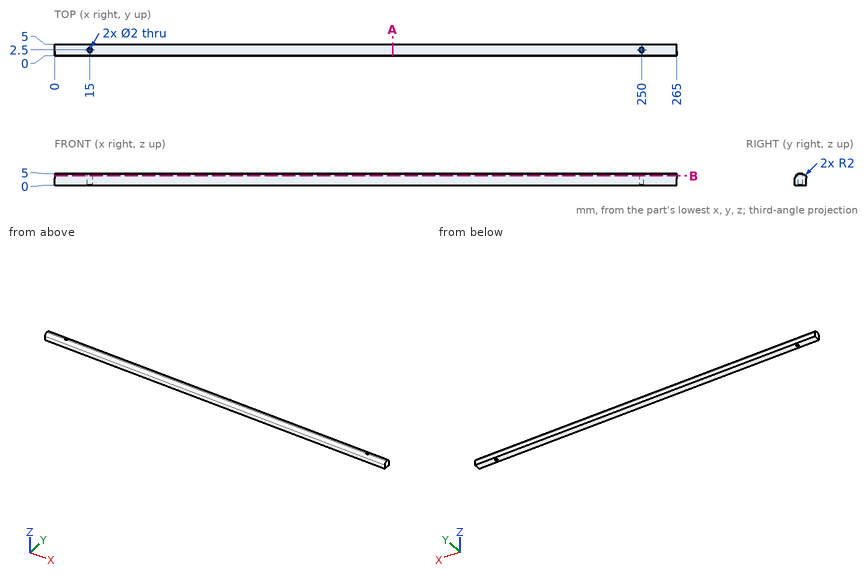
Study the drawing (mm; zero at the part's minimum x, y, z) and answer. Round coordinates to 2 decimals unless told otherwise and drop trailing zeros. Write each loop counter-clockwise with the first axis right and the second up, starting at its lowest first coordinate (ties: lowest second). Pieces come first, ordered by that corner, then holes. Notation, with made-up numbers: (15.5, 55.25) - (40.5, 55.25) arc R17 cw to (40.5, 65.25) - close; hole circle Ø7 at (56.25, 84.5). An arc over 180 degrees is marked (long way). Use CSV: the item, a comma, the result in double quotes.
Q1. Find section B-B, the plane z = 4.1. Write down the section's boundary in (x, y).
Values:
outline,"(0, 0.33) - (265, 0.33) - (265, 4.67) - (0, 4.67) - close; hole circle Ø2 at (15, 2.5); hole circle Ø2 at (250, 2.5)"
Q2. Find section A-A, the plane x = 144. Write down the section's boundary in (y, z), then the cut area to 3 significant figures.
Values:
outline,"(0, 0) - (5, 0) - (5, 3) arc R2 ccw to (3, 5) - (2, 5) arc R2 ccw to (0, 3) - close"
area,"23.3 mm²"
Q3. Straight lines are drawn through the part: line 1 along X through (y, z) = (1.95, 1.15); line 2 along Y through (x, z) = (250, 2.75); line 3 along X through (y, z) = (2.65, 0.8). For each, find the intervals that lie inside material, in ascending order.
Values:
line 1,"x = 0 to 14.16, 15.84 to 249.16, 250.84 to 265"
line 2,"y = 0 to 1.5, 3.5 to 5"
line 3,"x = 0 to 14.01, 15.99 to 249.01, 250.99 to 265"
